Can you work these out from the model? Positions are in its coordinate system, mm. A direction names the side the tool comes from. Coordinates: 2 decimals unless noted, no trailing zeros. Order: outer loops, then holes, each group sorted by start corner. A loop starts at its lowest first (then second) coordinate and runs counter-clockwise, first axis right, second up. Notation, with made-up numbers: (-12.5, -11) -> (8.5, -11) arc R11 cw to (8.5, 1) -> close; hole circle Ø7 at (38, -31). An arc over 180 degrees is marked (long way). Answer as a JSON object with one key per item and string values. Group by question number.
(1) I need wall thicknesses on line 1 (Z direction, x = -126, y = 5.5); line 2 (Y direction, x = -207.5, z = -24.5); line 3 (Y direction, x = -159, z = -9). Which ranges of each line are inside material? Lowest first, please.
(2) If we mould it in two halves opening along X, with no side actions, what happens to faces 5 (the flat face through (-118, 0, -26)), 6 (the cylindrical face through (-165, 10, 0)), 7 (the flat face through (0, 10, -4)), 8 (the cylindrical face through (-5, 10, 0))? For each: pulls with the +X half, pulls with the -X half, needs draft (parallel to the pull), parting line crosses it, or undercut.
(3) I want a section at B-B, the plane x = -16.5. List the corners of the cut face in (y, z) for me.
(4) For pin 1 (1 mm diameter, centred on x = -18, y = 10, fed in from +Z); pin 2 (1.3 mm diameter, centred on x = -57, y = 10, fed in from -Z); pin 3 (12 mm diameter, centred on x = -185.5, z = 3, fed in from -Y), each with a flat end and sliding along its axis, tell me the tip position at first contact or that it passes through.
(5) I want a section at A-A, the plane z = 0. List the corners of the cut face in (x, y) for me.
(6) Which directions (+Z, -Z, +X, -X, +Y, -Y) give clear straight access to the entire face, cutting with the end or side of a thin tool? Please do faces 1 (the flat face through (-118, 4, 18.8)), 2 (the cylindrical face through (-115, 10, 0)), 3 (the flat face through (-118, -1.2, -25)), 4 (the flat face through (-118, 5, 20)).
from build123d import *

# Parameters (mm, degrees)
BOSS_EXTRUDE1_DEPTH = 240
CUT_EXTRUDE1_DEPTH  = 243.165232847


with BuildPart() as part:
    # Sketch1 → Boss-Extrude1 (new body)
    with BuildSketch(Plane(origin=(0, 0, 0), x_dir=(0, 0, -1), z_dir=(1, 0, 0))):
        with BuildLine():
            Line((-21.2, 0), (-30, 0))
            Line((-30, 0), (-30, -1.2))
            Line((-30, -1.2), (-20, -1.2))
            ThreePointArc((-20, -1.2), (-19.151471863, -0.848528137), (-18.8, 0))
            Line((-18.8, 0), (-18.8, 8.4))
            ThreePointArc((-18.8, 8.4), (-18.448528137, 9.248528137), (-17.6, 9.6))
            Line((-17.6, 9.6), (17.6, 9.6))
            ThreePointArc((17.6, 9.6), (18.448528137, 9.248528137), (18.8, 8.4))
            Line((18.8, 8.4), (18.8, 0))
            ThreePointArc((18.8, 0), (19.151471863, -0.848528137), (20, -1.2))
            Line((20, -1.2), (30, -1.2))
            Line((30, -1.2), (30, 0))
            Line((30, 0), (21.2, 0))
            ThreePointArc((21.2, 0), (20.351471863, 0.351471863), (20, 1.2))
            Line((20, 1.2), (20, 9.6))
            ThreePointArc((20, 9.6), (19.648528137, 10.448528137), (18.8, 10.8))
            Line((18.8, 10.8), (-18.8, 10.8))
            ThreePointArc((-18.8, 10.8), (-19.648528137, 10.448528137), (-20, 9.6))
            Line((-20, 9.6), (-20, 1.2))
            ThreePointArc((-20, 1.2), (-20.351471863, 0.351471863), (-21.2, 0))
        make_face()
    extrude(amount=-BOSS_EXTRUDE1_DEPTH)

    # Sketch2 → Cut-Extrude1 (cut, through all)
    with BuildSketch(Plane(origin=(0, 10.8, 0), x_dir=(1, 0, 0), z_dir=(0, 1, 0))):
        with BuildLine():
            Line((-230, 5), (-210, 5))
            ThreePointArc((-210, 5), (-205, 0), (-210, -5))
            Line((-210, -5), (-230, -5))
            ThreePointArc((-230, -5), (-235, 0), (-230, 5))
        make_face()
        with BuildLine():
            Line((-190, 5), (-170, 5))
            ThreePointArc((-170, 5), (-165, 0), (-170, -5))
            Line((-170, -5), (-190, -5))
            ThreePointArc((-190, -5), (-195, 0), (-190, 5))
        make_face()
        with BuildLine():
            Line((-150, 5), (-130, 5))
            ThreePointArc((-130, 5), (-125, 0), (-130, -5))
            Line((-130, -5), (-150, -5))
            ThreePointArc((-150, -5), (-155, 0), (-150, 5))
        make_face()
        with BuildLine():
            Line((-110, 5), (-90, 5))
            ThreePointArc((-90, 5), (-85, 0), (-90, -5))
            Line((-90, -5), (-110, -5))
            ThreePointArc((-110, -5), (-115, 0), (-110, 5))
        make_face()
        with BuildLine():
            Line((-70, 5), (-50, 5))
            ThreePointArc((-50, 5), (-45, 0), (-50, -5))
            Line((-50, -5), (-70, -5))
            ThreePointArc((-70, -5), (-75, 0), (-70, 5))
        make_face()
        with BuildLine():
            Line((-30, 5), (-10, 5))
            ThreePointArc((-10, 5), (-5, 0), (-10, -5))
            Line((-10, -5), (-30, -5))
            ThreePointArc((-30, -5), (-35, 0), (-30, 5))
        make_face()
    extrude(amount=-CUT_EXTRUDE1_DEPTH, mode=Mode.SUBTRACT)


solid = part.part
Computed values:
{
 "1": {"line 1": "z = -20 to -18.8, 18.8 to 20", "line 2": "y = -1.2 to 0", "line 3": "y = 9.6 to 10.8"},
 "2": {"face 5": "needs draft", "face 6": "undercut", "face 7": "pulls with the +X half", "face 8": "undercut"},
 "3": {"outline": "(-1.2, -30) -> (0, -30) -> (0, -21.2) arc R1.2 cw to (1.2, -20) -> (9.6, -20) arc R1.2 ccw to (10.8, -18.8) -> (10.8, -5) -> (9.6, -5) -> (9.6, -17.6) arc R1.2 cw to (8.4, -18.8) -> (0, -18.8) arc R1.2 ccw to (-1.2, -20) -> close; (-1.2, 20) arc R1.2 ccw to (0, 18.8) -> (8.4, 18.8) arc R1.2 cw to (9.6, 17.6) -> (9.6, 5) -> (10.8, 5) -> (10.8, 18.8) arc R1.2 ccw to (9.6, 20) -> (1.2, 20) arc R1.2 cw to (0, 21.2) -> (0, 30) -> (-1.2, 30) -> close"},
 "4": {"pin 1": "stops at z = 20", "pin 2": "stops at z = -20", "pin 3": "stops at y = 9.6"},
 "5": {"outline": "(-240, 9.6) -> (-235, 9.6) -> (-235, 10.8) -> (-240, 10.8) -> close; (-205, 9.6) -> (-195, 9.6) -> (-195, 10.8) -> (-205, 10.8) -> close; (-165, 9.6) -> (-155, 9.6) -> (-155, 10.8) -> (-165, 10.8) -> close; (-125, 9.6) -> (-115, 9.6) -> (-115, 10.8) -> (-125, 10.8) -> close; (-85, 9.6) -> (-75, 9.6) -> (-75, 10.8) -> (-85, 10.8) -> close; (-45, 9.6) -> (-35, 9.6) -> (-35, 10.8) -> (-45, 10.8) -> close; (-5, 9.6) -> (0, 9.6) -> (0, 10.8) -> (-5, 10.8) -> close"},
 "6": {"face 1": "+X, -X, -Y", "face 2": "+Y, -Y", "face 3": "+Z, -Z, +X, -X, -Y", "face 4": "+Z, +X, -X, +Y"}
}
